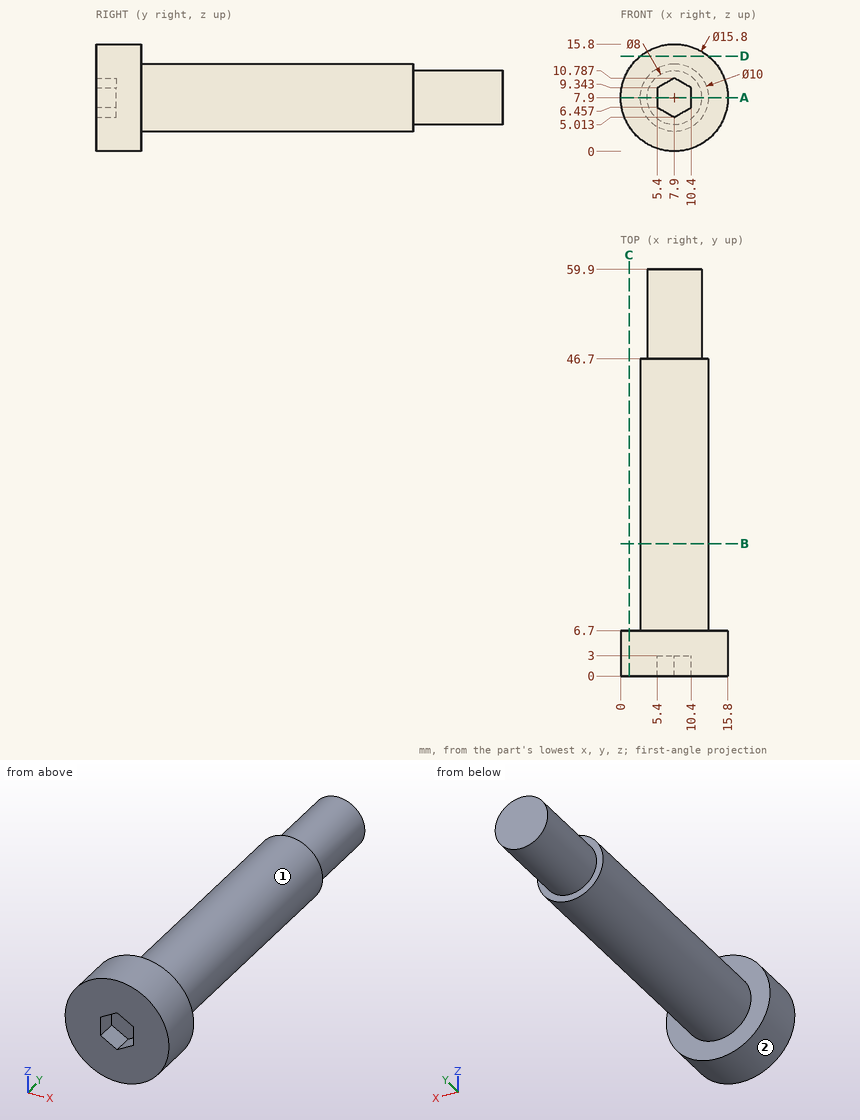
Study the drawing (mm; zero at the part's minimum x, y, z) and answer. A direction names the side the tool comes from. Coordinates: 2 decimals unless noted, no trailing zeros. Write each loop counter-clockwise with the first axis right and the second up, starting at its lowest first coordinate (ties: lowest second). Pieces come first, ordered by that corner, then holes. Notation, with made-up numbers: (74, 11) -> (110, 11) arc R23 cw to (110, 35) -> close; hole circle Ø11 at (68, 40). An arc over 180 degrees is marked (long way). Write each question's results on one line, items separated by ' | '. Start each with the question number.
1) A cutting plane is placed at C-C (x = 1.25). Determine the outline of the cut face in (y, z) (1 decimal).
2) A tool of negligible diameter and unlimited length cuts with its end or side. For the marked faces 1 and 2, from which of +Z, -Z, +X, -X, +Y, -Y can it reach the whole face along a straight path? Write none if from no direction.
3) A cutting plane is placed at B-B (y = 19.5). Determine the outline of the cut face in (x, z).
4) A cutting plane is placed at A-A (z = 7.9). Determine the outline of the cut face in (x, y).
5) Straight lines are drawn through the part: probe 1 along Y at (x, z) = (9.25, 15.25); probe 2 along Y at (x, z) = (3.25, 6.75); probe 3 along Z at (x, y) = (8, 53.5). For each, find the intervals that lie inside material, in ascending order.
6) A cutting plane is placed at D-D (z = 14). Determine the outline of the cut face in (x, y).
7) Flat-ended cylindrical pins translate along their axes: pin 1 Ø1 at (y, z) = (11.5, 10) entering from +X; pin 2 Ø2.5 at (x, z) = (8, 8) entering from -Y; pin 3 Ø4 at (y, z) = (10.5, 7) entering from -X. Find the tip coordinate at first contact, or state that the pin passes through.
Values follow:
1) outline: (0, 3.6) -> (6.7, 3.6) -> (6.7, 12.2) -> (0, 12.2) -> close
2) face 1: +Y | face 2: +Y, -Y
3) outline: circle Ø10 at (7.9, 7.9)
4) outline: (0, 0) -> (5.4, 0) -> (5.4, 3) -> (10.4, 3) -> (10.4, 0) -> (15.8, 0) -> (15.8, 6.7) -> (12.9, 6.7) -> (12.9, 46.7) -> (11.9, 46.7) -> (11.9, 59.9) -> (3.9, 59.9) -> (3.9, 46.7) -> (2.9, 46.7) -> (2.9, 6.7) -> (0, 6.7) -> close
5) probe 1: 0 to 6.7 | probe 2: 0 to 46.7 | probe 3: 3.9 to 11.9
6) outline: (2.88, 0) -> (12.92, 0) -> (12.92, 6.7) -> (2.88, 6.7) -> close
7) pin 1: x = 12.64 | pin 2: y = 3 | pin 3: x = 2.9
